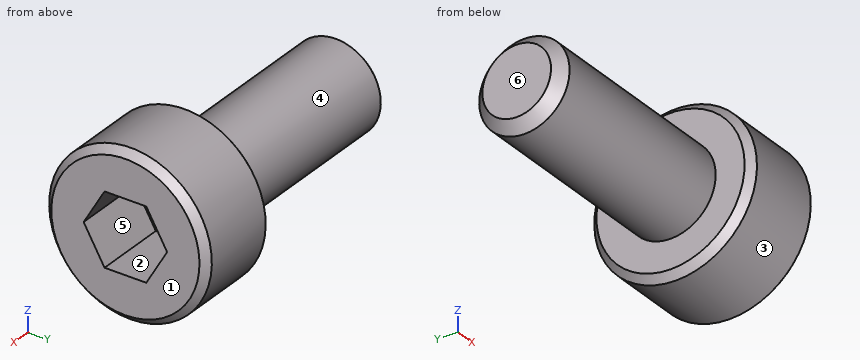
```python
from build123d import *

# Parameters (mm, degrees)
SKETCH1_W          = 6
SKETCH1_H          = 1.25
CUT_EXTRUDE1_DEPTH = 2
CHAMFER1_SIZE      = 0.2
CHAMFER2_SIZE      = 0.3


with BuildPart() as part:
    # Sketch1 → Revolve1 (revolve)
    with BuildSketch(Plane(origin=(0, 0, 0), x_dir=(1, 0, 0), z_dir=(0, 1, 0))):
        with Locations((-3, -0.625)):
            Rectangle(SKETCH1_W, SKETCH1_H)
        Polygon((0, 1), (0, 0), (0, -1.25), (2.5, -1.25), (2.5, 1), align=None)
    revolve(axis=Axis((0, 0, 1.25), (-1, 0, 0)))

    # Sketch3 → Cut-Extrude1 (cut)
    with BuildSketch(Plane(origin=(2.5, 0, 0), x_dir=(0, 0, -1), z_dir=(1, 0, 0))):
        Polygon((-1.25, 1.154700538), (-2.25, 0.577350269), (-2.25, -0.577350269), (-1.25, -1.154700538), (-0.25, -0.577350269), (-0.25, 0.577350269), align=None)
    extrude(amount=-CUT_EXTRUDE1_DEPTH, mode=Mode.SUBTRACT)

    # Chamfer1
    chamfer1_edges = [part.edges().sort_by_distance(p)[0] for p in [
        (0, 0, 3.5),
        (2.5, 0, 3.5),
    ]]
    chamfer(chamfer1_edges, length=CHAMFER1_SIZE)

    # Chamfer2
    chamfer2_edges = [part.edges().sort_by_distance(p)[0] for p in [
        (-6, 0, 2.5),
    ]]
    chamfer(chamfer2_edges, length=CHAMFER2_SIZE)


solid = part.part
```
Read the model definition and answer for the solid it produces. Units are mm, in the model's axes. Face numbers are marked on the shaded views. A direction names the side the tool comes from. Coordinates: 2 decimals unless noted, no trailing zeros. Write each loop counter-clockwise with the first axis right and the second up, starting at its lowest first coordinate (ties: lowest second). Pieces come first, ordered by that corner, then holes. Notation, with made-up numbers: (-15, -28.5) - (17, -28.5) arc R28 cw to (17, 10.5) - close; hole circle Ø9 at (-3, 24.5). An arc over 180 degrees is marked (long way). Answer as a JSON object with one key per item and string values. Group by question number.
1. Consider L1, parallel to X at y = 1.5, z = 2.2; L2, parallel to X at y = -0.1, z = 0.9; L3, parallel to Y at x = -2.5, z = 1.6. Determine where each line is inside the solid, lowest interval first. Write a range as [from, to].
2. The mould has two halves that part along Y. Classify the marked faces 1, 2 and 3: +Y half, -Y half, draft (parallel to the pull), parting line (faces both ways), or undercut.
3. A cutting plane is placed at A-A (y = 0). Determine the outline of the cut face in (x, z), plus the area to 3 significant figures.
4. Each of these flat-tipped pins is pushed along its axis until it touches: P1, Ø1.5, axis at x = 1, z = 2.5, coming from the -Y side; P2, Ø1.5, axis at y = 0.5, z = -0.5, coming from the -X side. Where does it stop, or does it pass through?
5. Which of the six approach directions +Z, -Z, +X, -X, +Y, -Y give full straight-line access (tool end or side, diameter ignored) to the marked faces 4, 5 and 6?
6. A cutting plane is placed at B-B (x = -2.75). Determine the outline of the cut face in (y, z), plus the area to 3 significant figures.
Worked out:
{
 "1": {"L1": "x = [0, 2.5]", "L2": "x = [-6, 0.5]", "L3": "y = [-1.2, 1.2]"},
 "2": {"face 1": "draft", "face 2": "undercut", "face 3": "parting line"},
 "3": {"outline": "(-6, 0.3) - (-5.7, 0) - (0, 0) - (0, -0.8) - (0.2, -1) - (2.3, -1) - (2.5, -0.8) - (2.5, 0.25) - (0.5, 0.25) - (0.5, 2.25) - (2.5, 2.25) - (2.5, 3.3) - (2.3, 3.5) - (0.2, 3.5) - (0, 3.3) - (0, 2.5) - (-5.7, 2.5) - (-6, 2.2) - close", "area": "22.1 mm²"},
 "4": {"P1": "stops at y = -2.19", "P2": "stops at x = -5.88"},
 "5": {"face 4": "-X", "face 5": "+X", "face 6": "+Z, -Z, -X, +Y, -Y"},
 "6": {"outline": "circle Ø2.5 at (0, 1.25)", "area": "4.91 mm²"}
}
